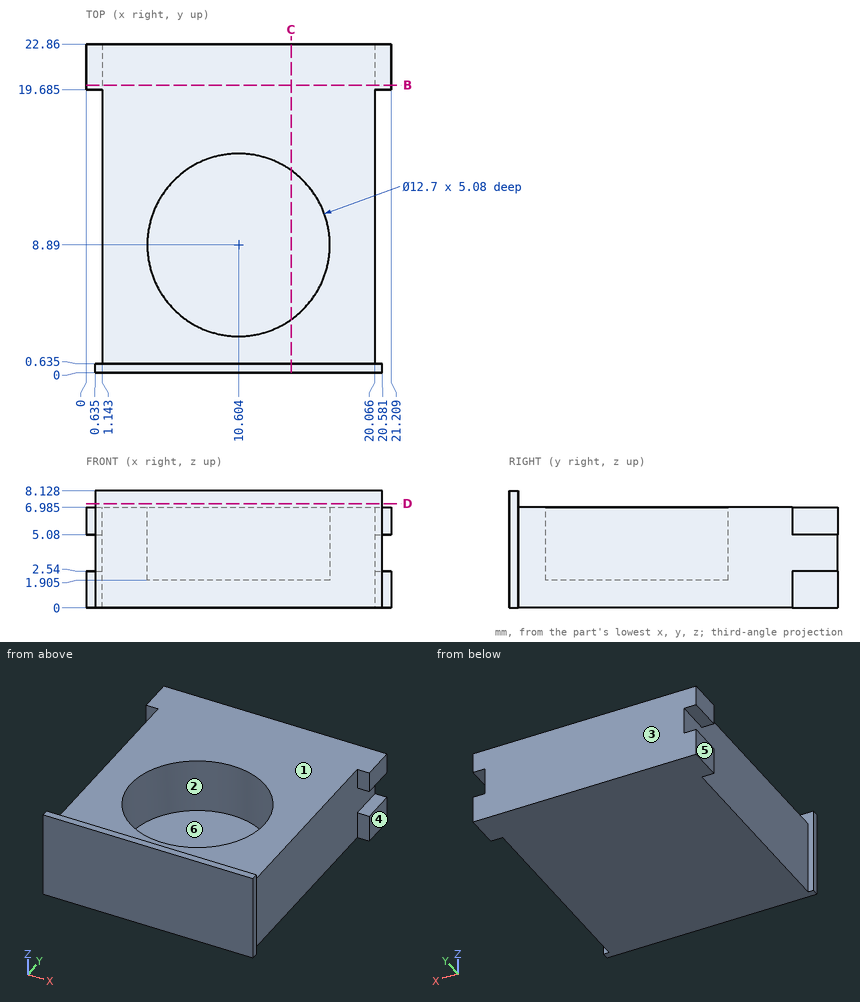
Can you work these out from the drawing? Everything is in mm from the part's minimum corner. A direction names the side the tool comes from. Round coordinates to 2 decimals unless told otherwise and drop trailing zeros. Loops run counter-clockwise (first coordinate to the right, second up) from the corner with the lowest first, then second, coordinate; pieces in that order, holes last.
1. If we section it at C-C on x = 14.25: Write out the boundary of the cut face in (y, z) (1 decimal), plus the area to 3 significant figures.
Answer list:
outline: (0, 0) - (22.9, 0) - (22.9, 7) - (14.1, 7) - (14.1, 1.9) - (3.7, 1.9) - (3.7, 7) - (0.6, 7) - (0.6, 8.1) - (0, 8.1) - close
area: 108 mm2
2. If we section it at D-D on z = 7.25: Write out the boundary of the cut face in (x, y) (1 decimal).
Answer list:
outline: (0.6, 0) - (20.6, 0) - (20.6, 0.6) - (0.6, 0.6) - close
3. If we section it at B-B on y = 20: Write out the boundary of the cut face in (x, z) (1 decimal), plus the area to 3 significant figures.
Answer list:
outline: (0, 0) - (21.2, 0) - (21.2, 2.5) - (20.1, 2.5) - (20.1, 5.1) - (21.2, 5.1) - (21.2, 7) - (0, 7) - (0, 5.1) - (1.1, 5.1) - (1.1, 2.5) - (0, 2.5) - close
area: 142 mm2
4. Which directions (+Z, -Z, +X, -X, +Y, -Y) give clear straight access to the entire face, cutting with the end or side of a thin tool? Please do the marked faces 1, 2 and 3.
Answer list:
face 1: +Z, +X, -X, +Y
face 2: +Z
face 3: +Z, -Z, +X, -X, +Y
5. If I drill on line 1 along X through (y, z) = (9, 3.5) (1 decimal); line 2 along Y through (x, z) = (9.5, 6); line 3 along Z through (x, y) = (13.75, 9) (1 decimal), over which ranges is the centre line in solid material (lowest first)?
Answer list:
line 1: x = 1.1 to 4.3, 17 to 20.1
line 2: y = 0 to 2.64, 15.14 to 22.86
line 3: z = 0 to 1.9
6. We'd pull the mould along X, two halves only. Please class the marked faces 4, 5 and 6: +X half, -X half, draft (parallel to the pull), parting line (faces both ways), or undercut.
Answer list:
face 4: +X half
face 5: -X half
face 6: undercut
7. For P1, Ø1.3, axis at x = 20.5, y = 21.5, coming from the +Z side (1 decimal); P2, Ø0.6, axis at x = 0.5, z = 5.5, coming from the -Y side; P3, Ø3.5, axis at y = 13.5, z = 4.5, coming from the -X side; P4, Ø0.7, axis at y = 0.5, z = 2.5, coming from the -X side (1 decimal), each with a flat end and sliding along its axis, tell me the tip position at first contact or that it passes through.
Answer list:
P1: stops at z = 7
P2: stops at y = 0
P3: stops at x = 1.14
P4: stops at x = 0.6
